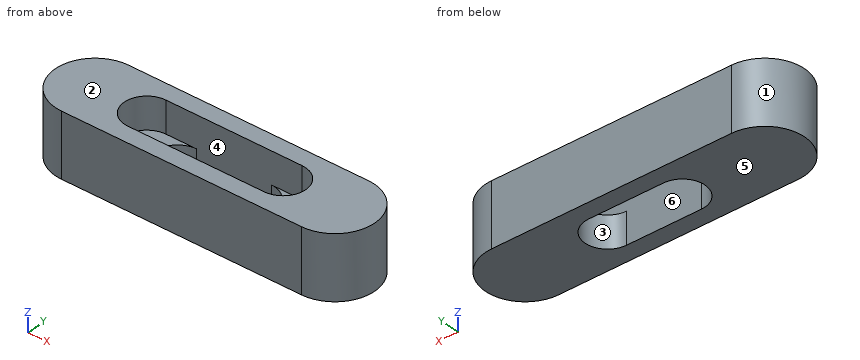
from build123d import *

# Parameters (mm, degrees)
F1_DEPTH = 12.7
F3_DEPTH = 12.7


with BuildPart() as f1:
    # F0 (on Top) → F1 (new body)
    with BuildSketch(Plane.XY):
        with BuildLine():
            Line((-47.625, -15.875), (47.625, -15.875))
            ThreePointArc((47.625, -15.875), (63.5, 0), (47.625, 15.875))
            Line((47.625, 15.875), (-47.625, 15.875))
            ThreePointArc((-47.625, 15.875), (-63.5, 0), (-47.625, -15.875))
        make_face()
        with BuildLine():
            ThreePointArc((27.051, 9.017), (36.068, 0), (27.051, -9.017))
            Line((27.051, -9.017), (-27.051, -9.017))
            ThreePointArc((-27.051, -9.017), (-36.068, 0), (-27.051, 9.017))
            Line((-27.051, 9.017), (27.051, 9.017))
        make_face(mode=Mode.SUBTRACT)
    extrude(amount=F1_DEPTH)

    # F2 (on face) → F3 (join)
    with BuildSketch(Plane(origin=(0, 0, 0), x_dir=(1, 0, 0), z_dir=(0, 0, -1))):
        with BuildLine():
            ThreePointArc((47.625, -15.875), (63.5, 0), (47.625, 15.875))
            Line((47.625, 15.875), (-47.625, 15.875))
            ThreePointArc((-47.625, 15.875), (-63.5, 0), (-47.625, -15.875))
            Line((-47.625, -15.875), (47.625, -15.875))
        make_face()
        with BuildLine():
            Line((27.051, -9.017), (14.859, -9.017))
            Line((14.859, -9.017), (-14.859, -9.017))
            Line((-14.859, -9.017), (-27.051, -9.017))
            ThreePointArc((-27.051, -9.017), (-36.068, 0), (-27.051, 9.017))
            Line((-27.051, 9.017), (-14.859, 9.017))
            Line((-14.859, 9.017), (14.859, 9.017))
            Line((14.859, 9.017), (27.051, 9.017))
            ThreePointArc((27.051, 9.017), (36.068, 0), (27.051, -9.017))
        make_face(mode=Mode.SUBTRACT)
        with BuildLine():
            Line((-27.051, -9.017), (-14.859, -9.017))
            ThreePointArc((-14.859, -9.017), (-23.876, 0), (-14.859, 9.017))
            Line((-14.859, 9.017), (-27.051, 9.017))
            ThreePointArc((-27.051, 9.017), (-36.068, 0), (-27.051, -9.017))
        make_face()
        with BuildLine():
            ThreePointArc((14.859, 9.017), (23.876, 0), (14.859, -9.017))
            Line((14.859, -9.017), (27.051, -9.017))
            ThreePointArc((27.051, -9.017), (36.068, 0), (27.051, 9.017))
            Line((27.051, 9.017), (14.859, 9.017))
        make_face()
    extrude(amount=F3_DEPTH)


solid = f1.part
Verification items for the finished model (mm, model axes). Face numbers are marked on the shaded views. A direction names the side the tool comes from. Coordinates: 2 decimals unless noted, no trailing zeros. Order: outer loops, then holes, each group sorted by start corner. A loop starts at its lowest first (then second) coordinate and runs counter-clockwise, first axis right, second up. Notation, with made-up numbers: M 10.5,-3.5 L 33.5,-3.5 A30 ccw 33.5,26.5 Z; hole C 7.5,10 d1. An arc over 180 degrees is marked long. Return JSON: item names as keys, results as strings.
1) Cross-section at A-A, the plane y = 0. Record the boundary of the cut face in (x, z).
Answer list:
{"outline": "M -63.5,-12.7 L -23.88,-12.7 L -23.88,0 L -36.07,0 L -36.07,12.7 L -63.5,12.7 Z; M 23.88,-12.7 L 63.5,-12.7 L 63.5,12.7 L 36.07,12.7 L 36.07,0 L 23.88,0 Z"}
2) Cross-section at B-B, the plane x = -13.5. Record the boundary of the cut face in (y, z) (3 decimals).
Answer list:
{"outline": "M -15.875,-12.7 L -9.017,-12.7 L -9.017,12.7 L -15.875,12.7 Z; M 9.017,-12.7 L 15.875,-12.7 L 15.875,12.7 L 9.017,12.7 Z"}
3) Release check for a two-part mould opening along X. For the marked faces 1, 2, 3 and 4 record: +X half, -X half, draft (parallel to the pull), parting line (faces both ways), or undercut.
Answer list:
{"face 1": "-X half", "face 2": "draft", "face 3": "undercut", "face 4": "undercut"}
4) Gauge pin test, flat ends, axial feed: pin 1 (1 mm diameter, centred on x = 26.5, y = -4.5, fed in from +Z); pin 2 (5 mm diameter, centred on y = 1, z = -2, fed in from +X); pin 3 (4 mm diameter, centred on y = 9.5, z = 3, fed in from -X). Record the tip position at first contact, or that the pin passes through.
Answer list:
{"pin 1": "z = 0", "pin 2": "x = 63.5", "pin 3": "x = -61.62"}
5) Access from +Z, -Z, +X, -X, +Y, -Y to the whole of each face (thin tool, end or side, straight path). Record for the marked faces 5 and 6.
Answer list:
{"face 5": "-Z, +X, -X, +Y, -Y", "face 6": "+Z"}
6) Cross-section at C-C, the plane z = -2. Record the boundary of the cut face in (x, y) (3 decimals), and give its area (3 significant figures).
Answer list:
{"outline": "M -47.625,-15.875 L 47.625,-15.875 A15.875 ccw 47.625,15.875 L -47.625,15.875 A15.875 ccw Z; hole M -14.859,-9.017 L 14.859,-9.017 A9.017 ccw 14.859,9.017 L -14.859,9.017 A9.017 ccw Z", "area": "3,020 mm2"}
7) Thickness scan on L1, parallel to Y at x = -15, z = 0.5 (3 decimals); L2, parallel to X at y = -7.5, z = -6.5; L3, parallel to X at y = 7, z = 4.5. Record the ranges inside material, lowest first. Write a range as [from, to].
Answer list:
{"L1": "[-15.875, -9.017], [9.017, 15.875]", "L2": "[-61.62, -19.86], [19.86, 61.62]", "L3": "[-61.87, -32.73], [32.73, 61.87]"}
8) Cross-section at D-D, the plane y = 10.5. Record the boundary of the cut face in (x, z), and give its area (3 significant figures).
Answer list:
{"outline": "M -59.53,-12.7 L 59.53,-12.7 L 59.53,12.7 L -59.53,12.7 Z", "area": "3,020 mm2"}
